Design review of the part built by this model. Coordinates are the model's own, in mm. Face numbers are marked on the shaded views. A direction names the side the tool comes from. Round coordinates to 2 decimals unless told otherwise and drop trailing zeros. Write each loop counter-clockwise with the first axis right and the second up, starting at its lowest first coordinate (ties: lowest second). Pieces come first, ordered by that corner, then holes. Notation, with made-up numbers: M 1.5,-8 L 12.5,-8 A6 cw 12.5,-2 Z; hole C 62,9 d1. An arc over 180 degrees is marked long. Use CSV: the item, a comma, the result in double quotes.
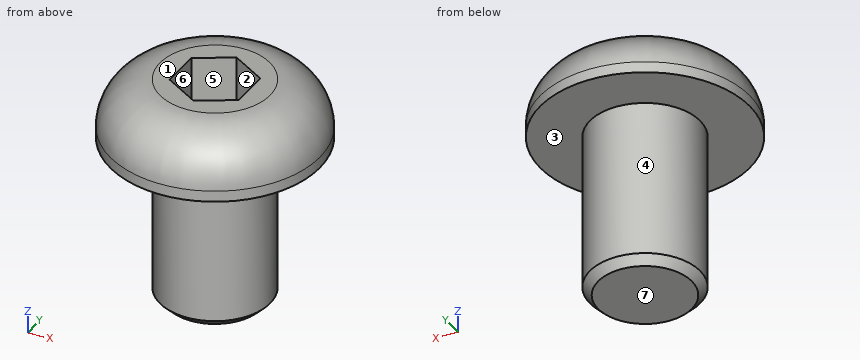
from build123d import *

# Parameters (mm, degrees)
SKETCH1_R           = 3.8
BOSS_EXTRUDE1_DEPTH = 2.2
SKETCH2_R           = 2
BOSS_EXTRUDE2_DEPTH = 6
CHAMFER1_SIZE       = 0.3
CUT_EXTRUDE1_DEPTH  = 2
FILLET1_R           = 1.8


with BuildPart() as part:
    # Sketch1 → Boss-Extrude1 (new body)
    with BuildSketch(Plane.XY):
        Circle(SKETCH1_R)
    extrude(amount=BOSS_EXTRUDE1_DEPTH)

    # Sketch2 → Boss-Extrude2 (add)
    with BuildSketch(Plane(origin=(0, 0, 0), x_dir=(-1, 0, 0), z_dir=(0, 0, -1))):
        Circle(SKETCH2_R)
    extrude(amount=BOSS_EXTRUDE2_DEPTH)

    # Chamfer1
    chamfer1_edges = [part.edges().sort_by_distance(p)[0] for p in [
        (2, 0, -6),
    ]]
    chamfer(chamfer1_edges, length=CHAMFER1_SIZE)

    # Sketch3 → Cut-Extrude1 (cut)
    with BuildSketch(Plane.XY.offset(2.2)):
        Polygon((0, 1.443375673), (-1.25, 0.721687836), (-1.25, -0.721687836), (0, -1.443375673), (1.25, -0.721687836), (1.25, 0.721687836), align=None)
    extrude(amount=-CUT_EXTRUDE1_DEPTH, mode=Mode.SUBTRACT)

    # Fillet1
    fillet1_edges = [part.edges().sort_by_distance(p)[0] for p in [
        (-3.8, 0, 2.2),
    ]]
    fillet(fillet1_edges, radius=FILLET1_R)


solid = part.part
1) For pin 1 Ø2 at (x, z) = (-0.5, -4.5) entering from +Y; pin 2 Ø3 at (y, z) = (-1, -3) entering from +X; pin 3 Ø2 at (x, y) = (-3, 1.5) entering from -Z, all flat-tipped, find the tip position at first contact; note any pin that passes through.
Answers:
pin 1,"y = 2"
pin 2,"x = 2"
pin 3,"z = 0"
2) The part is to be moulded in two halves that separate along X. For the marked faces 4, 5, 6 and 7, say which applies: released by +X, released by -X, zero draft, split by the parting line, or undercut.
Answers:
face 4,"split by the parting line"
face 5,"undercut"
face 6,"undercut"
face 7,"zero draft"
3) Add section B-B on z = 1.25. Write out the cut boundary in (x, y), then the cut area to 3 significant figures.
Answers:
outline,"C 0,0 d7.17; hole M -1.25,-0.72 L 0,-1.44 L 1.25,-0.72 L 1.25,0.72 L 0,1.44 L -1.25,0.72 Z"
area,"35.0 mm²"
4) Add section C-C on z = -0.25. Write out the cut boundary in (x, y), then the cut area to 3 significant figures.
Answers:
outline,"C 0,0 d4"
area,"12.6 mm²"
5) Add section A-A on y = 0. Write out the cut boundary in (x, z), then the cut area to 3 significant figures.
Answers:
outline,"M -3.8,0 L -2,0 L -2,-5.7 L -1.7,-6 L 1.7,-6 L 2,-5.7 L 2,0 L 3.8,0 L 3.8,0.4 A1.8 ccw 2,2.2 L 1.25,2.2 L 1.25,0.2 L -1.25,0.2 L -1.25,2.2 L -2,2.2 A1.8 ccw -3.8,0.4 Z"
area,"34.2 mm²"
6) Wall thickness on line 1 along Y through (x, z) = (-0.5, 1); line 2 along X through (y, z) = (-0.25, 1.5); line 3 along Z through (x, y) = (-0.25, -0.5): over which ranges is each line inside the solid? List them lowest first. Write a range as [from, to].
Answers:
line 1,"[-3.66, -1.15], [1.15, 3.66]"
line 2,"[-3.42, -1.25], [1.25, 3.42]"
line 3,"[-6, 0.2]"
7) Machinability: for the marked faces 1, 2 and 3, which of the approach directions +Z, -Z, +X, -X, +Y, -Y give a long, thin tool a straight path to every point of the face, cutting with its end or side? Answer none if there is none.
Answers:
face 1,"+Z, +X, -X, +Y, -Y"
face 2,"+Z"
face 3,"-Z"
